from build123d import *

# Parameters (mm, degrees)
F1_R      = 1.75
F1_R_2    = 3.35
F2_DEPTH  = 2
F3_R      = 2
F4_R      = 1.75
F4_R_2    = 3.35
F5_DEPTH  = 16.51
F6_SIZE2  = 2.8
F6_SIZE   = 1.6
F7_R      = 2.5
F7_R_2    = 1.4
F8_DEPTH  = 6.85
F9_W      = 20
F9_H      = 4
F10_DEPTH = 10.001
F11_W     = 20
F11_H     = 4
F12_DEPTH = 10.001
F13_W     = 10
F13_H     = 4
F14_DEPTH = 2.001
F15_W     = 20
F15_H     = 8
F16_DEPTH = 6
F17_W     = 18
F17_H     = 4
F18_DEPTH = 8
F19_R     = 1
F21_DEPTH = 0.2


with BuildPart() as f2:
    # F1 (on Top) → F2 (new body)
    with BuildSketch(Plane.XY):
        with BuildLine():
            ThreePointArc((8, 73.58), (2.343146, 71.236854), (0, 65.58))
            Line((0, 65.58), (0, 8))
            ThreePointArc((0, 8), (2.343146, 2.343146), (8, 0))
            Line((8, 0), (66.34, 0))
            ThreePointArc((66.34, 0), (71.996854, 2.343146), (74.34, 8))
            Line((74.34, 8), (74.34, 65.58))
            ThreePointArc((74.34, 65.58), (71.996854, 71.236854), (66.34, 73.58))
            Line((66.34, 73.58), (64.34, 73.58))
            Line((64.34, 73.58), (64.34, 59.98))
            Line((64.34, 59.98), (21.181552, 59.98))
            ThreePointArc((21.181552, 59.98), (20.280164, 59.811845), (19.500034, 59.33))
            ThreePointArc((19.500034, 59.33), (17.939776, 58.36631), (16.137, 58.03))
            Line((16.137, 58.03), (10, 58.03))
            Line((10, 58.03), (10, 73.58))
            Line((10, 73.58), (8, 73.58))
        make_face()
        with Locations((5, 12)):
            Circle(F1_R, mode=Mode.SUBTRACT)
        with Locations((5, 19)):
            Circle(F1_R_2, mode=Mode.SUBTRACT)
        with Locations((69.34, 12)):
            Circle(F1_R, mode=Mode.SUBTRACT)
        with Locations((69.34, 19)):
            Circle(F1_R_2, mode=Mode.SUBTRACT)
        with Locations((5, 54.58)):
            Circle(F1_R_2, mode=Mode.SUBTRACT)
        with Locations((5, 61.58)):
            Circle(F1_R, mode=Mode.SUBTRACT)
        with Locations((69.34, 54.58)):
            Circle(F1_R_2, mode=Mode.SUBTRACT)
        with Locations((69.34, 61.58)):
            Circle(F1_R, mode=Mode.SUBTRACT)
    extrude(amount=-F2_DEPTH)

    # F3
    f3_edges = [f2.edges().sort_by_distance(p)[0] for p in [
        (10, 58.03, -1),
        (64.34, 59.98, -1),
    ]]
    fillet(f3_edges, radius=F3_R)

    # F4 (on face) → F5 (join)
    with BuildSketch(Plane.XY):
        with BuildLine():
            ThreePointArc((8, 73.58), (2.343146, 71.236854), (0, 65.58))
            Line((0, 65.58), (0, 8))
            ThreePointArc((0, 8), (2.343146, 2.343146), (8, 0))
            Line((8, 0), (66.34, 0))
            ThreePointArc((66.34, 0), (71.996854, 2.343146), (74.34, 8))
            Line((74.34, 8), (74.34, 65.58))
            ThreePointArc((74.34, 65.58), (71.996854, 71.236854), (66.34, 73.58))
            Line((66.34, 73.58), (64.34, 73.58))
            Line((64.34, 73.58), (64.34, 2))
            Line((64.34, 2), (10, 2))
            Line((10, 2), (10, 73.58))
            Line((10, 73.58), (8, 73.58))
        make_face()
        with Locations((5, 12)):
            Circle(F4_R, mode=Mode.SUBTRACT)
        with Locations((5, 19)):
            Circle(F4_R_2, mode=Mode.SUBTRACT)
        with Locations((69.34, 12)):
            Circle(F4_R, mode=Mode.SUBTRACT)
        with Locations((69.34, 19)):
            Circle(F4_R_2, mode=Mode.SUBTRACT)
        with Locations((5, 54.58)):
            Circle(F4_R_2, mode=Mode.SUBTRACT)
        with Locations((5, 61.58)):
            Circle(F4_R, mode=Mode.SUBTRACT)
        with Locations((69.34, 54.58)):
            Circle(F4_R_2, mode=Mode.SUBTRACT)
        with Locations((69.34, 61.58)):
            Circle(F4_R, mode=Mode.SUBTRACT)
    extrude(amount=F5_DEPTH)

    # F6
    f6_edges = [f2.edges().sort_by_distance(p)[0] for p in [
        (3.25, 61.58, -2),
        (3.25, 12, -2),
        (67.59, 12, -2),
        (67.59, 61.58, -2),
    ]]
    chamfer(f6_edges, length=F6_SIZE, length2=F6_SIZE2)

    # F7 (on face) → F8 (join)
    with BuildSketch(Plane.XY):
        with Locations((37.17, 53.45)):
            Circle(F7_R)
        with Locations((37.17, 53.45)):
            Circle(F7_R_2, mode=Mode.SUBTRACT)
        with Locations((37.17, 20.13)):
            Circle(F7_R)
        with Locations((37.17, 20.13)):
            Circle(F7_R_2, mode=Mode.SUBTRACT)
    extrude(amount=F8_DEPTH)

    # F9 (on face) → F10 (cut, through all)
    with BuildSketch(Plane.YZ.offset(10)):
        with Locations((36.79, 2)):
            Rectangle(F9_W, F9_H)
    extrude(amount=-F10_DEPTH, mode=Mode.SUBTRACT)

    # F11 (on face) → F12 (cut, through all)
    with BuildSketch(Plane(origin=(64.34, 0, 0), x_dir=(0, -1, 0), z_dir=(-1, 0, 0))):
        with Locations((-36.79, 2)):
            Rectangle(F11_W, F11_H)
    extrude(amount=-F12_DEPTH, mode=Mode.SUBTRACT)

    # F13 (on face) → F14 (cut, through all)
    with BuildSketch(Plane(origin=(0, 2, 0), x_dir=(-1, 0, 0), z_dir=(0, 1, 0))):
        with Locations((-50.755, 2)):
            Rectangle(F13_W, F13_H)
        with Locations((-23.585, 2)):
            Rectangle(F13_W, F13_H)
    extrude(amount=-F14_DEPTH, mode=Mode.SUBTRACT)

    # F15 (on face) → F16 (join)
    with BuildSketch(Plane.XY):
        with Locations((54.34, 55.98)):
            Rectangle(F15_W, F15_H)
    extrude(amount=F16_DEPTH)

    # F17 (on face) → F18 (cut, through all)
    with BuildSketch(Plane(origin=(0, 59.98, 0), x_dir=(-1, 0, 0), z_dir=(0, 1, 0))):
        with Locations((-55.34, 2)):
            Rectangle(F17_W, F17_H)
    extrude(amount=-F18_DEPTH, mode=Mode.SUBTRACT)

    # F19
    f19_edges = [f2.edges().sort_by_distance(p)[0] for p in [
        (46.34, 55.98, 4),
        (44.34, 55.98, 6),
    ]]
    fillet(f19_edges, radius=F19_R)

    # F20 (on face) → F21 (join)
    with BuildSketch(Plane(origin=(0, 0, -2), x_dir=(1, 0, 0), z_dir=(0, 0, -1))):
        with BuildLine():
            ThreePointArc((8, 2), (0.928932, -0.928932), (-2, -8))
            Line((-2, -8), (-2, -65.58))
            ThreePointArc((-2, -65.58), (0.928932, -72.651068), (8, -75.58))
            Line((8, -75.58), (12, -75.58))
            Line((12, -75.58), (12, -61.98))
            Line((12, -61.98), (62.34, -61.98))
            Line((62.34, -61.98), (62.34, -75.58))
            Line((62.34, -75.58), (66.34, -75.58))
            ThreePointArc((66.34, -75.58), (73.411068, -72.651068), (76.34, -65.58))
            Line((76.34, -65.58), (76.34, -8))
            ThreePointArc((76.34, -8), (73.411068, -0.928932), (66.34, 2))
            Line((66.34, 2), (8, 2))
        make_face()
        with BuildLine():
            Line((0, -65.58), (0, -8))
            ThreePointArc((0, -8), (2.343146, -2.343146), (8, 0))
            Line((8, 0), (66.34, 0))
            ThreePointArc((66.34, 0), (71.996854, -2.343146), (74.34, -8))
            Line((74.34, -8), (74.34, -65.58))
            ThreePointArc((74.34, -65.58), (71.996854, -71.236854), (66.34, -73.58))
            Line((66.34, -73.58), (64.34, -73.58))
            Line((64.34, -73.58), (64.34, -61.98))
            ThreePointArc((64.34, -61.98), (63.754214, -60.565786), (62.34, -59.98))
            Line((62.34, -59.98), (21.181552, -59.98))
            ThreePointArc((21.181552, -59.98), (20.280164, -59.811845), (19.500034, -59.33))
            ThreePointArc((19.500034, -59.33), (17.939776, -58.36631), (16.137, -58.03))
            Line((16.137, -58.03), (12, -58.03))
            ThreePointArc((12, -58.03), (10.585786, -58.615786), (10, -60.03))
            Line((10, -60.03), (10, -73.58))
            Line((10, -73.58), (8, -73.58))
            ThreePointArc((8, -73.58), (2.343146, -71.236854), (0, -65.58))
        make_face(mode=Mode.SUBTRACT)
    extrude(amount=-F21_DEPTH)


solid = f2.part
CAD build for the part. Positions are in the model's coordinates, mm. A direction names the side the tool comes from. Round coordinates to 2 decimals unless told otherwise and drop trailing zeros. Write each loop counter-clockwise with the first axis right and the second up, starting at its lowest first coordinate (ties: lowest second). Pieces come first, ordered by that corner, then holes.
(1) 3-axis set-ups, long thin cutter, end or side, ignore diameter. For faces 4 (the face through (35.77, 53.51, 3.38)), 5 (the face through (46.34, 56, 1)), 6 (the face through (45.755, 1, 2)), 7 (the face through (10.6, 58.6, -0.9)): which of +Z, -Z, +X, -X, +Y, -Y reach the whole face in a straight line?
(2) Mould opens along X. For faces 1 (the face through (74.34, 36, 7)), 2 (the face through (55, 56, 6)), 3 (the face through (64.34, 38, 9)) say: pulls with the +X half, pulls with the -X half, needs draft (parallel to the pull), parting line crosses it, or undercut.
(3) Slice it at A-A, the plane y = 12. Write the cut outline in (x, z), and give its area (3 significant figures).
(4) Slice it at B-B, the plane x = 69.34. Count the separate pieces of the cut face and the enclosed holes in it, and give its area (3 significant figures).
(5) Probe line 1 along Y through (x, z) = (37.17, 2.25); line 2 along Z through (x, y) = (64.5, 43); line 3 along Y through (x, z) = (5, 6.5). List the from-to ranges inside material, lowest first.
(6) Slice it at D-D, the plane x = 53. Write the cut outline in (y, z).
(7) Drop flat-ended pins along their axis: P1, Ø8, axis at x = 22.5, z = 1, coming from the +Y side; P2, Ø2, axis at x = 70, z = 2.5, coming from the -Y side; P3, Ø1.5, axis at y = 32, z = 6.5, coming from the -X side; P4, Ø1, axis at x = 49.5, z = 1, coming from the -Y side. Give the stop position or say it passes through.
From the geometry:
1. face 4: +Z
1. face 5: +Y, -Y
1. face 6: -Y
1. face 7: +Z, +Y
2. face 1: pulls with the +X half
2. face 2: undercut
2. face 3: undercut
3. outline: (-2, -2) - (1.65, -2) - (3.25, 0.8) - (3.25, 16.51) - (0, 16.51) - (0, -1.8) - (-2, -1.8) - close; (6.75, 0.8) - (8.35, -2) - (65.99, -2) - (67.59, 0.8) - (67.59, 16.51) - (64.34, 16.51) - (64.34, 0) - (10, 0) - (10, 16.51) - (6.75, 16.51) - close; (71.09, 0.8) - (72.69, -2) - (76.34, -2) - (76.34, -1.8) - (74.34, -1.8) - (74.34, 16.51) - (71.09, 16.51) - close
3. area: 341 mm2
4. separate pieces: 5
4. enclosed holes: 1
4. area: 875 mm2
5. line 1: y = 0 to 2, 17.63 to 18.73, 21.53 to 22.63, 50.95 to 52.05, 54.85 to 55.95
5. line 2: z = -2 to 0, 4 to 16.51
5. line 3: y = 0.58 to 10.25, 13.75 to 15.65, 22.35 to 51.23, 57.93 to 59.83, 63.33 to 73
6. outline: (-2, -2) - (61.98, -2) - (61.98, -1.8) - (59.98, -1.8) - (59.98, 0) - (0, 0) - (0, -1.8) - (-2, -1.8) - close; (0, 4) - (2, 4) - (2, 16.51) - (0, 16.51) - close; (51.98, 4) - (59.98, 4) - (59.98, 6) - (51.98, 6) - close
7. P1: stops at y = 61.98
7. P2: stops at y = 0.46
7. P3: stops at x = 0
7. P4: passes through
